For this review, take the finished solid that the model builds, in its own axes (mm). A direction names the side the tool comes from. Round coordinates to 2 decimals unless told otherwise and drop trailing zeros. Order: outer loops, then holes, each group sorted by start corner. A loop starts at its lowest first (then second) coordinate and runs counter-clockwise, first axis right, second up. Notation, with made-up numbers: (-21.5, -22.75) - (26.5, -22.75) arc R22 ccw to (26.5, -0.75) - close; hole circle Ø2 at (-9.75, 13). An arc over 180 degrees is marked (long way). One line per item, written item: value.
```python
from build123d import *

# Parameters (mm, degrees)
SKETCH_2_R          = 8
SKETCH_2_R_2        = 1.75
EXTRUDE_1_DEPTH     = 4
CUT_EXTRUDE_START   = -0.5
CUT_EXTRUDE_1_DEPTH = 0.5


with BuildPart() as part:
    # 草图2 → 凸台-拉伸1 (new body)
    with BuildSketch(Plane(origin=(0, 0, 0), x_dir=(1, 0, 0), z_dir=(0, 1, 0))):
        with BuildLine():
            Line((-13, 10), (-13, -10))
            ThreePointArc((-13, -10), (-12.121320344, -12.121320344), (-10, -13))
            Line((-10, -13), (10, -13))
            ThreePointArc((10, -13), (12.121320344, -12.121320344), (13, -10))
            Line((13, -10), (13, 10))
            ThreePointArc((13, 10), (12.121320344, 12.121320344), (10, 13))
            Line((10, 13), (-10, 13))
            ThreePointArc((-10, 13), (-12.121320344, 12.121320344), (-13, 10))
        make_face()
        with Locations(Location((0, 0, 0), (0, 0, 270))):
            Circle(SKETCH_2_R, mode=Mode.SUBTRACT)
        with Locations(Location((-10, 10, 0), (0, 0, 270))):
            Circle(SKETCH_2_R_2, mode=Mode.SUBTRACT)
        with Locations(Location((10, 10, 0), (0, 0, 270))):
            Circle(SKETCH_2_R_2, mode=Mode.SUBTRACT)
        with Locations(Location((10, -10, 0), (0, 0, 270))):
            Circle(SKETCH_2_R_2, mode=Mode.SUBTRACT)
        with Locations(Location((-10, -10, 0), (0, 0, 270))):
            Circle(SKETCH_2_R_2, mode=Mode.SUBTRACT)
    extrude(amount=EXTRUDE_1_DEPTH)

    # 草图3 → 切除-拉伸1 (cut)
    with BuildSketch(Plane(origin=(0, 4, 0), x_dir=(1, 0, 0), z_dir=(0, 1, 0)).offset(CUT_EXTRUDE_START)):
        with BuildLine():
            ThreePointArc((-8.088989369, -3.382202126), (-7.593724303, -3.503347811), (-7.110532834, -3.666104584))
            ThreePointArc((-7.110532834, -3.666104584), (-8, 0), (-7.110532834, 3.666104584))
            ThreePointArc((-7.110532834, 3.666104584), (-7.593724303, 3.503347811), (-8.088989369, 3.382202126))
            Line((-8.088989369, 3.382202126), (-13, 2.4))
            Line((-13, 2.4), (-13, -2.4))
            Line((-13, -2.4), (-8.088989369, -3.382202126))
        make_face()
        with BuildLine():
            ThreePointArc((-3.382202126, 8.088989369), (-3.503347811, 7.593724303), (-3.666104584, 7.110532834))
            ThreePointArc((-3.666104584, 7.110532834), (0, 8), (3.666104584, 7.110532834))
            ThreePointArc((3.666104584, 7.110532834), (3.503347811, 7.593724303), (3.382202126, 8.088989369))
            Line((3.382202126, 8.088989369), (2.4, 13))
            Line((2.4, 13), (-2.4, 13))
            Line((-2.4, 13), (-3.382202126, 8.088989369))
        make_face()
        with BuildLine():
            ThreePointArc((8, 0), (7.774453764, -1.886231339), (7.110532834, -3.666104584))
            ThreePointArc((7.110532834, -3.666104584), (7.593724303, -3.503347811), (8.088989369, -3.382202126))
            Line((8.088989369, -3.382202126), (13, -2.4))
            Line((13, -2.4), (13, 2.4))
            Line((13, 2.4), (8.088989369, 3.382202126))
            ThreePointArc((8.088989369, 3.382202126), (7.593724303, 3.503347811), (7.110532834, 3.666104584))
            ThreePointArc((7.110532834, 3.666104584), (7.774453764, 1.886231339), (8, 0))
        make_face()
        with BuildLine():
            Line((0, -13), (0, -8))
            ThreePointArc((0, -8), (-1.886231339, -7.774453764), (-3.666104584, -7.110532834))
            ThreePointArc((-3.666104584, -7.110532834), (-3.503347811, -7.593724303), (-3.382202126, -8.088989369))
            Line((-3.382202126, -8.088989369), (-2.4, -13))
            Line((-2.4, -13), (0, -13))
        make_face()
        with BuildLine():
            ThreePointArc((3.666104584, -7.110532834), (1.886231339, -7.774453764), (0, -8))
            Line((0, -8), (0, -13))
            Line((0, -13), (2.4, -13))
            Line((2.4, -13), (3.382202126, -8.088989369))
            ThreePointArc((3.382202126, -8.088989369), (3.503347811, -7.593724303), (3.666104584, -7.110532834))
        make_face()
    extrude(amount=CUT_EXTRUDE_1_DEPTH, mode=Mode.SUBTRACT)


solid = part.part
```
Item 1: The part is to be moulded in two halves that separate along X. For faces 3 (the flat face through (-8, 4, -8)), 4 (the flat face through (-2.884, 3.746, -10.579)), 5 (the cylindrical face through (-12.1, 1.97, -12.14)), say which applies: +X half, -X half, draft (parallel to the pull), parting line (faces both ways), or undercut.
Returned:
face 3: draft
face 4: undercut
face 5: -X half
Item 2: Take a section at D-D (x = 10.75). Write out the cut boundary in (y, z).
Returned:
outline: (0, -12.9) - (4, -12.9) - (4, -11.58) - (0, -11.58) - close; (0, -8.42) - (4, -8.42) - (4, -2.85) - (3.5, -2.85) - (3.5, 2.85) - (4, 2.85) - (4, 8.42) - (0, 8.42) - close; (0, 11.58) - (4, 11.58) - (4, 12.9) - (0, 12.9) - close
Item 3: Wall thickness on line 1 (X direction, y = 2.3, z = -10); line 2 (Z direction, x = 9, y = 3.25); line 3 (Z direction, x = -9.25, y = 3.35): over which ranges is each line inside the solid? List them lowest first.
Returned:
line 1: -13 to -11.75, -8.25 to 8.25, 11.75 to 13
line 2: -13 to -11.44, -8.56 to 8.56, 11.44 to 13
line 3: -13 to -11.58, -8.42 to 8.42, 11.58 to 13
Item 4: For P1, Ø2, axis at x = -10, z = -10, coming from the +Y side; P2, Ø3, axis at x = 9.5, z = 1, coming from the +Y side, all flat-tipped, find the tip position at first contact; note any pin that passes through.
Returned:
P1: through
P2: y = 3.5
Item 5: Take a section at B-B (x = 2). Write out the cut boundary in (y, z), plus the area to 3 significant figures.
Returned:
outline: (0, -13) - (3.5, -13) - (3.5, -7.75) - (0, -7.75) - close; (0, 7.75) - (3.5, 7.75) - (3.5, 13) - (0, 13) - close
area: 36.8 mm^2
Item 6: Take a section at C-C (y = 1.5). Write out the cut boundary in (x, z).
Returned:
outline: (-13, -10) arc R3 ccw to (-10, -13) - (10, -13) arc R3 ccw to (13, -10) - (13, 10) arc R3 ccw to (10, 13) - (-10, 13) arc R3 ccw to (-13, 10) - close; hole circle Ø3.5 at (-10, -10); hole circle Ø3.5 at (-10, 10); hole circle Ø16 at (0, 0); hole circle Ø3.5 at (10, -10); hole circle Ø3.5 at (10, 10)
Item 7: Machinability: for faces 1 (the flat face through (-10, 3.5, 0)), 2 (the flat face through (-6, 0, 6)), which of the approach directions +Z, -Z, +X, -X, +Y, -Y give a long, thin tool a straight path to every point of the face, cutting with its end or side? Answer none if there is none.
Returned:
face 1: +Y
face 2: +Z, -Z, +X, -X, -Y
Item 8: Take a section at A-A (z = 0). Write out the cut boundary in (x, y).
Returned:
outline: (-13, 0) - (-8, 0) - (-8, 3.5) - (-13, 3.5) - close; (8, 0) - (13, 0) - (13, 3.5) - (8, 3.5) - close
